from build123d import *

# Parameters (mm, degrees)
CROQUIS1_W              = 101.6
CROQUIS1_H              = 50.8
SALIENTE_EXTRUIR1_DEPTH = 6.31
CROQUIS2_R              = 4.7625
CORTAR_EXTRUIR1_DEPTH   = 6.31
CROQUIS3_R              = 5
CORTAR_EXTRUIR2_DEPTH   = 10


with BuildPart() as part:
    # Croquis1 → Saliente-Extruir1 (new body)
    with BuildSketch(Plane(origin=(0, 0, 0), x_dir=(1, 0, 0), z_dir=(0, 1, 0))):
        Rectangle(CROQUIS1_W, CROQUIS1_H)
    extrude(amount=SALIENTE_EXTRUIR1_DEPTH)

    # Croquis2 → Cortar-Extruir1 (cut)
    with BuildSketch(Plane(origin=(0, 6.31, 0), x_dir=(1, 0, 0), z_dir=(0, 1, 0))):
        with Locations(Location((-38.1, -12.7, 0), (0, 0, 270))):
            Circle(CROQUIS2_R)
        with Locations(Location((-12.7, 12.7, 0), (0, 0, 270))):
            Circle(CROQUIS2_R)
    extrude(amount=-CORTAR_EXTRUIR1_DEPTH, mode=Mode.SUBTRACT)

    # Croquis3 → Cortar-Extruir2 (cut)
    with BuildSketch(Plane(origin=(0, 6.31, 0), x_dir=(1, 0, 0), z_dir=(0, 1, 0))):
        with Locations(Location((25.4, 0, 0), (0, 0, 270))):
            Circle(CROQUIS3_R)
    extrude(amount=-CORTAR_EXTRUIR2_DEPTH, mode=Mode.SUBTRACT)


solid = part.part
Could you check a few things on this model? Use its own coordinates, in mm. Round coordinates to 2 decimals unless told otherwise and drop trailing zeros. Order: outer loops, then holes, each group sorted by start corner. A loop starts at its lowest first (then second) coordinate and runs counter-clockwise, first axis right, second up.
Q1. Imagine slicing it at A-A, the plane z = -12.7. List the corners of the cut face in (x, y) for me.
Geometry says:
outline: (-50.8, 0) - (-17.46, 0) - (-17.46, 6.31) - (-50.8, 6.31) - close; (-7.94, 0) - (50.8, 0) - (50.8, 6.31) - (-7.94, 6.31) - close
Q2. Please list where these lines run through material, in increasing order: probe 1 along X at (y, z) = (4.75, -12.7); probe 2 along X at (y, z) = (2, 12.7); probe 3 along Z at (x, y) = (23.5, 6).
Geometry says:
probe 1: x = -50.8 to -17.46, -7.94 to 50.8
probe 2: x = -50.8 to -42.86, -33.34 to 50.8
probe 3: z = -25.4 to -4.62, 4.62 to 25.4
Q3. Thinking about a two-plate mould opening in X: for faces 1 (the face through (-1, 0, 0)), 2 (the face through (30.357, 3.199, -0.651)), 3 (the face through (-50.8, 3, 0)), which applies, released by +X, released by -X, zero draft, split by the parting line, or undercut?
Geometry says:
face 1: zero draft
face 2: undercut
face 3: released by -X
Q4. Imagine slicing it at B-B, the plane x = -38.1. List the corners of the cut face in (y, z) for me.
Geometry says:
outline: (0, -25.4) - (6.31, -25.4) - (6.31, 7.94) - (0, 7.94) - close; (0, 17.46) - (6.31, 17.46) - (6.31, 25.4) - (0, 25.4) - close
Q5. Imagine slicing it at C-C, the plane y = 4.25. List the corners of the cut face in (x, z) for me (1 decimal), then the cut area to 3 significant figures.
Geometry says:
outline: (-50.8, -25.4) - (50.8, -25.4) - (50.8, 25.4) - (-50.8, 25.4) - close; hole circle Ø9.5 at (-38.1, 12.7); hole circle Ø9.5 at (-12.7, -12.7); hole circle Ø10 at (25.4, 0)
area: 4,940 mm2
Q6. I'm going to push flat-ended pins straight in: P1, Ø15, axis at x = -12.7, z = -12.7, coming from the +Y side; P2, Ø7.5, axis at x = -38.1, z = 12.7, coming from the +Y side. Where does each tip first touch, or does it pass through?
Geometry says:
P1: stops at y = 6.31
P2: passes through
